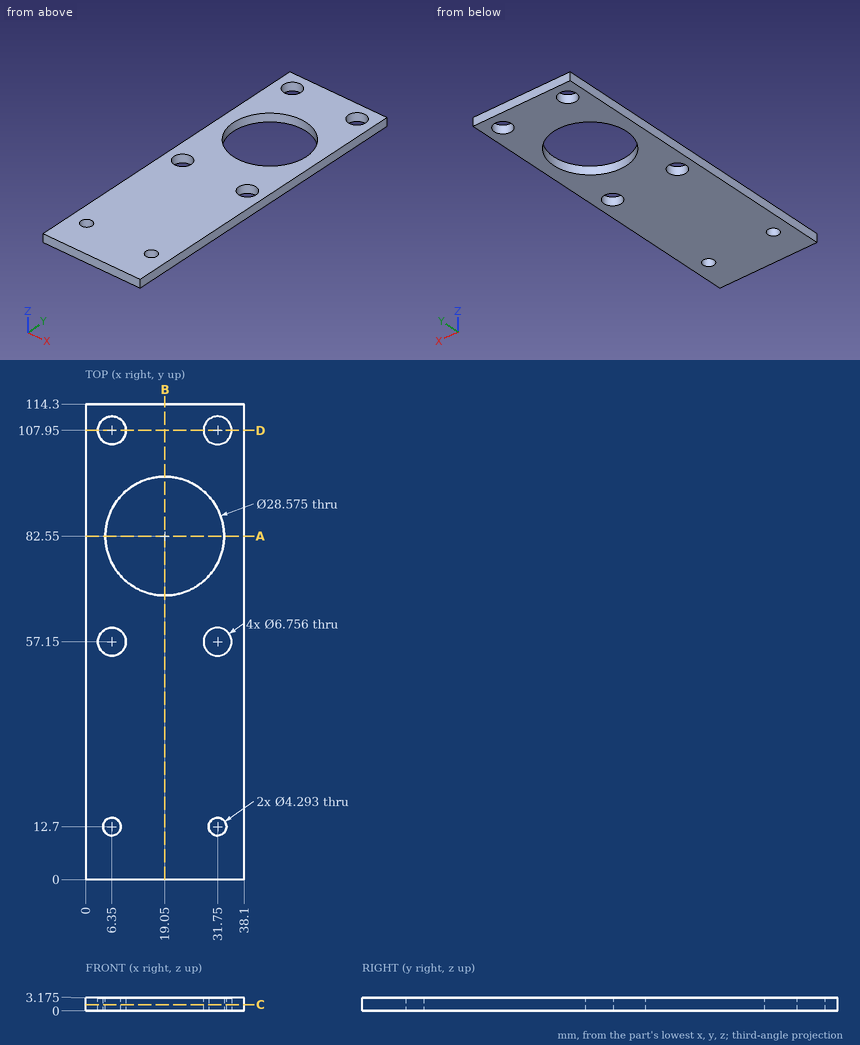
For this review, use the dimensioned drawing (mm, ordinates from the lowest corner) and the shaded views. Give positions to 0.01 mm unless a question says otherwise; leave off trailing zeros. Order: outer loops, then holes, each group sorted by start corner. A loop starts at its lowest first (then second) coordinate and runs counter-clockwise, first axis right, second up. Notation, with made-up numbers: (20.25, 18.5) - (53.25, 18.5) arc R13 cw to (53.25, 38.5) - close; hole circle Ø9 at (61, 80). An arc over 180 degrees is marked (long way). Use CSV: the item, a comma, the result in double quotes. Start each with the question number.
Q1. For P1, Ø5.5, axis at x = 31.75, y = 12.7, coming from the -Z side; P2, Ø6, axis at x = 31.75, y = 107.95, coming from the +Z side, all flat-tipped, find the tip position at first contact; note any pin that passes through.
Q2. Take a section at C-C (z = 1.45). Count the separate pieces of the cut face and the enclosed holes in it, and give its area (3 significant figures).
Q3. For line 1 (X direction, y = 12.7, z = 1.5); line 2 (Y direction, x = 31.5, z = 2.5) (1 decimal); line 3 (X direction, y = 56, z = 2), list the stretches that pass through material, from the lowest coordinate up.
Q4. Take a section at D-D (y = 107.95). State the section outline as (x, z) points (1 decimal).
Q5. Take a section at A-A (y = 82.55). State the section outline as (x, z) points (1 decimal).
Q6. Take a section at B-B (x = 19.05). State the section outline as (y, z) points (1 decimal).
Calculated:
1,P1,"stops at z = 0"
1,P2,"passes through"
2,separate pieces,"1"
2,enclosed holes,"7"
2,area,"3,540 mm²"
3,line 1,"x = 0 to 4.2, 8.5 to 29.6, 33.9 to 38.1"
3,line 2,"y = 0 to 10.6, 14.8 to 53.8, 60.5 to 75.5, 89.6 to 104.6, 111.3 to 114.3"
3,line 3,"x = 0 to 3.17, 9.53 to 28.57, 34.93 to 38.1"
4,outline,"(0, 0) - (3, 0) - (3, 3.2) - (0, 3.2) - close; (9.7, 0) - (28.4, 0) - (28.4, 3.2) - (9.7, 3.2) - close; (35.1, 0) - (38.1, 0) - (38.1, 3.2) - (35.1, 3.2) - close"
5,outline,"(0, 0) - (4.8, 0) - (4.8, 3.2) - (0, 3.2) - close; (33.3, 0) - (38.1, 0) - (38.1, 3.2) - (33.3, 3.2) - close"
6,outline,"(0, 0) - (68.3, 0) - (68.3, 3.2) - (0, 3.2) - close; (96.8, 0) - (114.3, 0) - (114.3, 3.2) - (96.8, 3.2) - close"
